Autodesk Inventor part; units mm, degrees
ref_plane "YZ Plane" through (0, 0, 0) normal (1, 0, 0) x (0, 1, 0)
ref_plane "XZ Plane" through (0, 0, 0) normal (0, 1, 0) x (-1, 0, 0)
ref_plane "XY Plane" through (0, 0, 0) normal (0, 0, 1) x (1, 0, 0)
sketch "Sketch1" plane through (0, 0, 0) normal (0, 0, 1) x (1, 0, 0)
  circle A0 centre (0, 0) radius 2.1844
  circle A1 centre (38.1, 0) radius 2.1844
  line L0 (0, 6.35) -> (38.1, 6.35)
  line L1 (38.1, -6.35) -> (0, -6.35)
  arc A2 (0, 6.35) -> (0, -6.35) centre (0, 0) ccw
  arc A3 (38.1, -6.35) -> (38.1, 6.35) centre (38.1, 0) ccw
  circle A4 centre (12.7, 0) radius 2.1844
  dimension "d0" = 4.3688
  dimension "d2" = 4.3688
  dimension "d8" = 4.3688
extrude "Extrusion1" add sketch "Sketch1" along normal blind 1.5875
properties part number "distancesensorcablemanage"
Here's how the part is built. I have some questions about the finished solid (model axes, mm). Give positions to 0.01 mm unless a question says otherwise; leave off trailing zeros. Order: outer loops, then holes, each group sorted by start corner. A loop starts at its lowest first (then second) coordinate and runs counter-clockwise, first axis right, second up. Notation, with made-up numbers: M 47.25,-26.5 L 85.25,-26.5 A10 ccw 85.25,-22.5 Z; hole C -19,83.5 d11. An arc over 180 degrees is marked long. Use a Markdown table: item, result. Add a question column.
1. Suppose I cut it at C-C (x = 12.7). List the corners of the cut face in (y, z) for me, and give its area (3 significant figures).
2. Suppose I cut it at A-A (y = 0). List the corners of the cut face in (x, z) for me, and give its area (3 significant figures).
3. Suppose I cut it at B-B (z = 0.3). List the corners of the cut face in (x, y) for me, and give its area (3 significant figures).
4. If we mould it in two halves opening along X, with no side actions, what happens to faces 1 (the cylindrical face through (40.118, 0.837, 0.783)), 2 (the flat face through (19, 0, 1.588)), 3 (the cylindrical face through (2.084, -0.656, 0.783)), 4 (the cylindrical face through (44.45, 0.14, 0.78))? For each: +X half, -X half, draft (parallel to the pull), parting line (faces both ways), or undercut.
5. Suppose I cut it at D-D (x = -1.5). List the corners of the cut face in (y, z) for me, and give its area (3 significant figures).
6. For pin 1 Ø3.5 at (x, y) = (0, 0) entering from +Z, with a flat end and sliding along its axis, tell me the tip position at first contact or that it passes through.
7. I need wall thicknesses on probe 1 along Y at (x, z) = (12.5, 0.3); probe 2 along X at (y, z) = (0.75, 0.5); probe 3 along Y at (x, z) = (14, 0.9). Which ranges of each line are inside material? Lowest first, please. Write a range as from..to.
Results list:
| question | item | result |
|---|---|---|
| 1 | outline | M -6.35,0 L -2.18,0 L -2.18,1.59 L -6.35,1.59 Z; M 2.18,0 L 6.35,0 L 6.35,1.59 L 2.18,1.59 Z |
| 1 | area | 13.2 mm² |
| 2 | outline | M -6.35,0 L -2.18,0 L -2.18,1.59 L -6.35,1.59 Z; M 2.18,0 L 10.52,0 L 10.52,1.59 L 2.18,1.59 Z; M 14.88,0 L 35.92,0 L 35.92,1.59 L 14.88,1.59 Z; M 40.28,0 L 44.45,0 L 44.45,1.59 L 40.28,1.59 Z |
| 2 | area | 59.8 mm² |
| 3 | outline | M 0,-6.35 L 38.1,-6.35 A6.35 ccw 38.1,6.35 L 0,6.35 A6.35 ccw Z; hole C 0,0 d4.37; hole C 12.7,0 d4.37; hole C 38.1,0 d4.37 |
| 3 | area | 566 mm² |
| 4 | face 1 | undercut |
| 4 | face 2 | draft |
| 4 | face 3 | undercut |
| 4 | face 4 | +X half |
| 5 | outline | M -6.17,0 L -1.59,0 L -1.59,1.59 L -6.17,1.59 Z; M 1.59,0 L 6.17,0 L 6.17,1.59 L 1.59,1.59 Z |
| 5 | area | 14.5 mm² |
| 6 | pin 1 | passes through |
| 7 | probe 1 | y = -6.35..-2.18, 2.18..6.35 |
| 7 | probe 2 | x = -6.31..-2.05, 2.05..10.65, 14.75..36.05, 40.15..44.41 |
| 7 | probe 3 | y = -6.35..-1.76, 1.76..6.35 |
